Input: part model. Units: mm. Frame: model coordinates. Give positions to 0.01 mm unless a question says otherwise; leave off trailing zeros. Loops run counter-clockwise (first coordinate to the right, second up) from the corner with the lowest first, then second, coordinate; pieces in that order, holes last. Notation, with made-up numbers: (15, -19.75) -> (51, -19.75) arc R31 cw to (51, 7.25) -> close; hole circle Ø7 at (40.5, -3.5). An arc over 180 degrees is marked (long way). Use CSV: the item, a comma, the result in double quotes.
```python
from build123d import *

# Parameters (mm, degrees)
F1_DEPTH = 1016
F3_DEPTH = 127.001
F5_DEPTH = 127.001


with BuildPart() as f1:
    # F0 (on Front) → F1 (new body)
    with BuildSketch(Plane.XZ):
        with BuildLine():
            Line((0, -127), (0, 0))
            Line((0, 0), (-50.8, 0))
            ThreePointArc((-50.8, 0), (-73.25064, -9.29936), (-82.55, -31.75))
            Line((-82.55, -31.75), (-82.55, -95.25))
            ThreePointArc((-82.55, -95.25), (-73.25064, -117.70064), (-50.8, -127))
            Line((-50.8, -127), (0, -127))
        make_face()
    extrude(amount=F1_DEPTH)

    # F2 (on face) → F3 (cut, through all)
    with BuildSketch(Plane.XY):
        Polygon((0, -82.003355), (0, 0), (-82.003355, 0), align=None)
    extrude(amount=-F3_DEPTH, mode=Mode.SUBTRACT)

    # F4 (on face) → F5 (cut, through all)
    with BuildSketch(Plane.XY):
        Polygon((0, -1016), (0, -793.203355), (-222.796645, -1016), align=None)
    extrude(amount=-F5_DEPTH, mode=Mode.SUBTRACT)


solid = f1.part
```
1) Section query D-D (y = -72.5). Return loops of the section in (x, z).
From the geometry:
outline,"(-82.55, -95.25) arc R31.75 ccw to (-50.8, -127) -> (-9.5, -127) -> (-9.5, 0) -> (-50.8, 0) arc R31.75 ccw to (-82.55, -31.75) -> close"
2) Section query B-B (z = -73). Return loops of the section in (x, y).
From the geometry:
outline,"(-82.55, -875.75) -> (0, -793.2) -> (0, -82) -> (-82, 0) -> (-82.55, 0) -> close"
3) Section query C-C (x = -36). Return loops of the section in (y, z).
From the geometry:
outline,"(-829.2, -127) -> (-46, -127) -> (-46, 0) -> (-829.2, 0) -> close"
4) Ray query, line 1 (Z direction, x = -53.5, y = -476.5); line 2 (X direction, y = -76, z = -104.5); line 3 (Y direction, x = -7.5, z = -101). Return the intervals inside material, ascending.
From the geometry:
line 1,"z = -126.88 to -0.12"
line 2,"x = -81.17 to -6"
line 3,"y = -800.7 to -74.5"
5) Section query A-A (y = -417.5). Return loops of the section in (x, z).
From the geometry:
outline,"(-82.55, -95.25) arc R31.75 ccw to (-50.8, -127) -> (0, -127) -> (0, 0) -> (-50.8, 0) arc R31.75 ccw to (-82.55, -31.75) -> close"
6) Contact query for a flat-ended pin moving along its axis: pin 1 (1 mm diameter, centred on x = -73, z = -46, fed in from +Y). Output: stop coordinate, or through.
From the geometry:
pin 1,"stops at y = -8.5"
